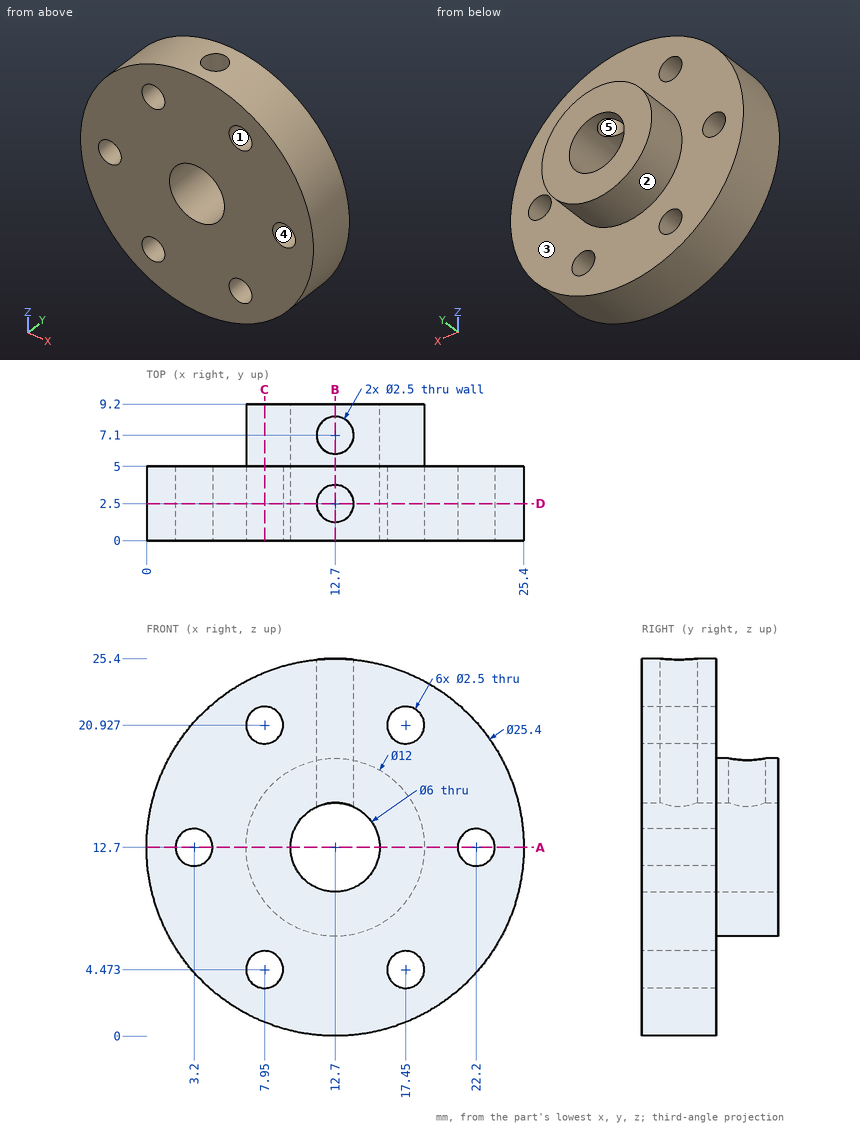
Can you work these out from the drawing? Everything is in mm from the part's minimum corner. A direction names the side the tool comes from. Give positions to 0.01 mm unless a question says otherwise; leave off trailing zeros. Write each loop counter-clockwise with the first axis right and the second up, starting at its lowest first coordinate (ties: lowest second). Pieces come first, ordered by that corner, then holes. Notation, with made-up numbers: M 64,55.5 L 104,55.5 A34 cw 104,91.5 Z; hole C 29,39 d5. An arc over 180 degrees is marked long. Answer in a Markdown table with one row per item. Add a question column.
Item 1: We'd pull the mould along Z, two halves only. Please class the marked faces 1, 2 and 3: released by +Z, released by -Z, zero draft, split by the parting line, or undercut.
Item 2: Imagine slicing it at A-A, the plane z = 12.7. Write out the boundary of the cut face in (x, y).
Item 3: Imagine slicing it at D-D, the plane y = 2.5. Write out the boundary of the cut face in (x, z).
Item 4: For pin 1 Ø1.5 at (x, z) = (17.45, 4.47) entering from -Y; pin 2 Ø3 at (x, y) = (12.7, 7.1) entering from +Z; pin 3 Ø4 at (x, z) = (3.2, 12.7) entering from +Y; pin 4 Ø1 at (y, z) = (3, 20.5) entering from +X, each with a flat end and sliding along its axis, tell me the tip position at first contact or that it passes through.
Item 5: Imagine slicing it at B-B, the plane x = 12.7. Write out the boundary of the cut face in (y, z).
Item 6: Please list where these lines run through material, in increasing order: L1, parallel to X at y = 2.5, z = 20.75; L2, parallel to X at y = 4.25, z = 5.25 (1 decimal); L3, parallel to X at y = 1, z = 5.5.
Item 7: On a 3-axis mill with a long thin cutter (end or side, diameter ignored), from which of +Z, -Z, +X, -X, +Y, -Y can I reach the whole of each face in a straight line? I mean the marked faces 4 and 5. Say none if no direction works.
Item 8: Imagine slicing it at C-C, the plane x = 7.95. Write out the boundary of the cut face in (y, z), plus the area to 3 significant figures.
Evaluation:
| question | item | result |
|---|---|---|
| 1 | face 1 | undercut |
| 1 | face 2 | split by the parting line |
| 1 | face 3 | zero draft |
| 2 | outline | M 0,0 L 1.95,0 L 1.95,5 L 0,5 Z; M 4.45,0 L 9.7,0 L 9.7,9.2 L 6.7,9.2 L 6.7,5 L 4.45,5 Z; M 15.7,0 L 20.95,0 L 20.95,5 L 18.7,5 L 18.7,9.2 L 15.7,9.2 Z; M 23.45,0 L 25.4,0 L 25.4,5 L 23.45,5 Z |
| 3 | outline | M 11.45,15.43 L 11.45,25.34 A12.7 ccw long 13.95,25.34 L 13.95,15.43 A3 cw long Z; hole C 3.2,12.7 d2.5; hole C 7.95,4.47 d2.5; hole C 7.95,20.93 d2.5; hole C 17.45,4.47 d2.5; hole C 17.45,20.93 d2.5; hole C 22.2,12.7 d2.5 |
| 4 | pin 1 | passes through |
| 4 | pin 2 | stops at z = 18.7 |
| 4 | pin 3 | stops at y = 5 |
| 4 | pin 4 | stops at x = 23.09 |
| 5 | outline | M 0,0 L 5,0 L 5,6.7 L 9.2,6.7 L 9.2,9.7 L 0,9.7 Z; M 0,15.7 L 1.25,15.7 L 1.25,25.4 L 0,25.4 Z; M 3.75,15.7 L 5.85,15.7 L 5.85,18.7 L 5,18.7 L 5,25.4 L 3.75,25.4 Z; M 8.35,15.7 L 9.2,15.7 L 9.2,18.7 L 8.35,18.7 Z |
| 6 | L1 | x = 2.88 to 6.71, 9.19 to 11.45, 13.95 to 16.21, 18.69 to 22.52 |
| 6 | L2 | x = 2.4 to 7, 8.9 to 16.5, 18.4 to 23 |
| 6 | L3 | x = 2.24 to 7.24, 8.66 to 16.74, 18.16 to 23.16 |
| 7 | face 4 | +Y, -Y |
| 7 | face 5 | +Z |
| 8 | outline | M 0,0.92 L 5,0.92 L 5,3.22 L 0,3.22 Z; M 0,5.72 L 5,5.72 L 5,9.03 L 9.2,9.03 L 9.2,16.37 L 5,16.37 L 5,19.68 L 0,19.68 Z; M 0,22.18 L 5,22.18 L 5,24.48 L 0,24.48 Z |
| 8 | area | 124 mm² |
